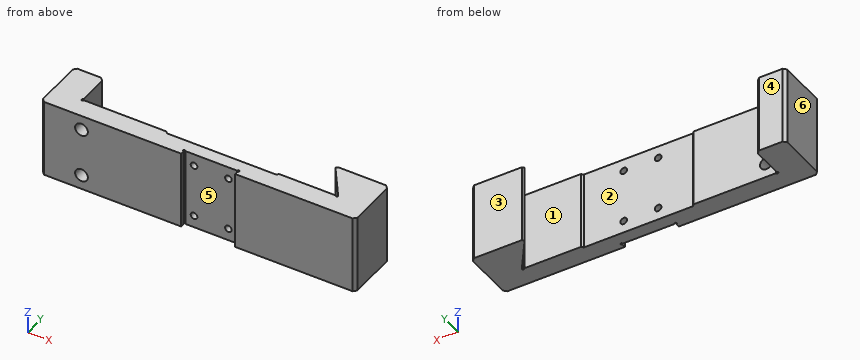
```python
from build123d import *
from OCP.BRepFilletAPI import BRepFilletAPI_MakeChamfer

# Parameters (mm, degrees)
EXTRUDE_1_DEPTH          = 40
CUT_EXTRUDE_1_DEPTH      = 335.402452144
CUT_EXTRUDE_1_DEPTH_BACK = 80
SKETCH_2_W               = 115
SKETCH_2_H               = 2
CHAMFER_1_SIZE           = 2
CUT_EXTRUDE_1_2_DEPTH    = 80
CUT_EXTRUDE_2_DEPTH      = 335.402452144
CUT_EXTRUDE_2_DEPTH_BACK = 80
SKETCH_4_W               = 55
SKETCH_4_H               = 5
CUT_EXTRUDE_2_2_DEPTH    = 80
HOLE_WIZARD_M8_1_D       = 6.8
HOLE_WIZARD_1_D          = 13
CHAMFER_2_SIZE           = 3
CHAMFER_2_SIZE2          = 2.154045129


with BuildPart() as part:
    # 草图1 → 凸台-拉伸1 (new, symmetric)
    with BuildSketch(Plane.XY):
        Polygon((0, 0), (0, 55), (30, 55), (30, 20), (290, 20), (265.492736163, 55), (320, 55), (320, 0), align=None)
    extrude(amount=EXTRUDE_1_DEPTH, both=True)

    # 草图2 → Cut-Extrude 1 (cut, two sides: drawn at the far end of the back side and taken through both)
    with BuildSketch(Plane.XY.offset(40).offset(-CUT_EXTRUDE_1_DEPTH_BACK)):
        with Locations((172.5, 19)):
            Rectangle(SKETCH_2_W, SKETCH_2_H)
    extrude(amount=CUT_EXTRUDE_1_DEPTH + CUT_EXTRUDE_1_DEPTH_BACK, mode=Mode.SUBTRACT)

    # 倒角1
    chamfer_1_edges = [part.edges().sort_by_distance(p)[0] for p in [
        (230, 18, 0),
        (115, 18, 0),
    ]]
    chamfer(chamfer_1_edges, length=CHAMFER_1_SIZE - 0.0001)  # a hair under: the kernel refuses the full size

    # 草图3 → Cut-Extrude 1 2 (cut)
    with BuildSketch(Plane.XY.offset(40)):
        Polygon((287.171572875, 20), (288.585786438, 18.585786438), (290, 20), (288.585786438, 21.414213562), align=None)
        Polygon((28.585786438, 20), (30, 21.414213562), (31.414213562, 20), (30, 18.585786438), align=None)
    extrude(amount=-CUT_EXTRUDE_1_2_DEPTH, mode=Mode.SUBTRACT)

    # 草图4 → Cut-Extrude 2 (cut, two sides: drawn at the far end of the back side and taken through both)
    with BuildSketch(Plane.XY.offset(40).offset(-CUT_EXTRUDE_2_DEPTH_BACK)):
        with Locations((170, 2.5)):
            Rectangle(SKETCH_4_W, SKETCH_4_H)
    extrude(amount=CUT_EXTRUDE_2_DEPTH + CUT_EXTRUDE_2_DEPTH_BACK, mode=Mode.SUBTRACT)

    # 草图5 → Cut-Extrude 2 2 (cut)
    with BuildSketch(Plane.XY.offset(40)):
        Polygon((198.914213562, 5), (197.5, 6.414213562), (196.085786438, 5), (197.5, 3.585786438), align=None)
    cut_extrude_2_2 = extrude(amount=-CUT_EXTRUDE_2_2_DEPTH, mode=Mode.SUBTRACT)

    # 镜向1: Cut-Extrude 2 2 across plane
    add(cut_extrude_2_2.mirror(Plane(origin=(170, 0, 0), x_dir=(0, 0, 1), z_dir=(1, 0, 0))), mode=Mode.SUBTRACT)

    # M8 螺纹孔1 (through all)
    with Locations(Plane.XZ):
        with Locations((152.5, 27.5), (187.5, 27.5), (187.5, -27.5), (152.5, -27.5)):
            Hole(HOLE_WIZARD_M8_1_D / 2)

    # 孔1 (through all)
    with Locations(Plane(origin=(0, 20, 0), x_dir=(1, 0, 0), z_dir=(0, 1, 0))):
        with Locations((41, 25), (41, -25)):
            Hole(HOLE_WIZARD_1_D / 2)

    # 倒角2: one chamfer whose edges measure the first distance from different faces: ONE call of the kernel's chamfer builder (chamfer() names one face for all edges)
    chamfer_2_edges_1 = [part.edges().sort_by_distance(p)[0] for p in [
        (0, 0, 0),
        (0, 55, 0),
        (30, 55, 0),
        (320, 55, 0),
        (320, 0, 0),
    ]]
    chamfer_2_edges_2 = [part.edges().sort_by_distance(p)[0] for p in [
        (265.492736163, 55, 0),
    ]]
    chamfer_2_side_2 = [part.faces().sort_by_distance(p)[0] for p in [
        (292.746368081, 55, 0),
    ]]
    chamfer_2 = BRepFilletAPI_MakeChamfer(part.part.solid().wrapped)
    for e in chamfer_2_edges_1:
        chamfer_2.Add(CHAMFER_2_SIZE, e.wrapped)
    for e in chamfer_2_edges_2:
        chamfer_2.Add(CHAMFER_2_SIZE, CHAMFER_2_SIZE2, e.wrapped, chamfer_2_side_2[0].wrapped)  # the first distance lies on this face
    add(Compound.cast(chamfer_2.Shape()), mode=Mode.REPLACE)


solid = part.part
```
Source: CAD feature listing. Evaluate the final solid. Frame: model axes, mm. Face numbers are marked on the shaded views. A direction names the side the tool comes from. Round coordinates to 2 decimals unless told otherwise and drop trailing zeros. Loops run counter-clockwise (first coordinate to the right, second up) from the corner with the lowest first, then second, coordinate; pieces in that order, holes last. Notation, with made-up numbers: M -33.75,67.5 L -4.75,67.5 A20 ccw -4.75,92.5 Z; hole C 62,-26 d9. An arc over 180 degrees is marked long. Use a Markdown table: item, result. Add a question column.
1. Cut plane D-D, the plane x = 274.5. Output: boundary loops of the cut face in (y, z), and give its area (3 significant figures).
2. Contact query for flat-ended pins moving along their axis: pin 1 (8 mm diameter, centred on x = 187.5, z = -27.5, fed in from -Y); pin 2 (3 mm diameter, centred on y = 1, z = 1.5, fed in from -X); pin 3 (5 mm diameter, centred on x = 138.5, z = -10.5, fed in from +Y). Output: stop coordinate, or through.
3. Cut plane B-B, the plane x = 41. Output: boundary loops of the cut face in (y, z), and give its area (3 significant figures).
4. Cut plane A-A, the plane y = 15. Output: boundary loops of the cut face in (x, z).
5. Pull-direction query (X, two-part tool) for the marked faces 4, 5 and 6; classes: +X half, -X half, draft (parallel to the pull), parting line (faces both ways), or undercut.
6. Cut plane C-C, the plane y = 38. Output: boundary loops of the cut face in (x, z), and give its area (3 significant figures).
7. Set-up query: the marked faces 1, 2 and 3. Return all of +Z, -Z, +X, -X, +Y, -Y with unobstructed straight access to the full face (end or side cutting, diameter ignored); none if empty.
8. Ray query, line 1 along Z through (x, y) = (41, 12); line 2 along Z through (x, y) = (187.5, 15); line 3 along X through (y, z) = (13, 27). Return the intervals inside material, ascending. Write a range as [from, to].
Solution:
| question | item | result |
|---|---|---|
| 1 | outline | M 0,-40 L 20,-40 L 20,40 L 0,40 Z; M 42.14,-40 L 55,-40 L 55,40 L 42.14,40 Z |
| 1 | area | 2,630 mm2 |
| 2 | pin 1 | stops at y = 5 |
| 2 | pin 2 | stops at x = 0.5 |
| 2 | pin 3 | stops at y = 18 |
| 3 | outline | M 0,-40 L 20,-40 L 20,-31.5 L 0,-31.5 Z; M 0,-18.5 L 20,-18.5 L 20,18.5 L 0,18.5 Z; M 0,31.5 L 20,31.5 L 20,40 L 0,40 Z |
| 3 | area | 1,080 mm2 |
| 4 | outline | M 0,-40 L 320,-40 L 320,40 L 0,40 Z; hole C 41,-25 d13; hole C 41,25 d13; hole C 152.5,-27.5 d6.8; hole C 152.5,27.5 d6.8; hole C 187.5,-27.5 d6.8; hole C 187.5,27.5 d6.8 |
| 5 | face 4 | draft |
| 5 | face 5 | undercut |
| 5 | face 6 | -X half |
| 6 | outline | M 0,-40 L 30,-40 L 30,40 L 0,40 Z; M 277.4,-40 L 320,-40 L 320,40 L 277.4,40 Z |
| 6 | area | 5,810 mm2 |
| 7 | face 1 | +Z, -Z |
| 7 | face 2 | +Z, -Z, +Y |
| 7 | face 3 | +Z, -Z, +X, -X, +Y |
| 8 | line 1 | z = [-40, -31.5], [-18.5, 18.5], [31.5, 40] |
| 8 | line 2 | z = [-40, -30.9], [-24.1, 24.1], [30.9, 40] |
| 8 | line 3 | x = [0, 34.82], [47.18, 149.14], [155.86, 184.14], [190.86, 320] |
